```python
from build123d import *

# Parameters (mm, degrees)
BOSS_EXTRUDE1_START = 62.8
SKETCH2_W           = 1.28
SKETCH2_H           = 0.8
BOSS_EXTRUDE1_DEPTH = 6.4
BOSS_EXTRUDE2_START = 65.6
SKETCH3_W           = 1.28
SKETCH3_H           = 6.4
BOSS_EXTRUDE2_DEPTH = 0.8
BOSS_EXTRUDE3_START = 65.2
SKETCH4_W           = 1.8
SKETCH4_H           = 0.9
BOSS_EXTRUDE3_DEPTH = 1.6


with BuildPart() as part:
    # Sketch1 → Revolve1 (revolve)
    with BuildSketch(Plane.XY.offset(66), mode=Mode.PRIVATE) as revolve1_sk:
        Polygon((-58.2, 20.3), (-59.4, 20.3), (-59.4, 18), (-61, 18), (-61, 23.6), (-60.6, 24), (-59.4, 24), (-59.4, 21), (-58.2, 21), align=None)
    revolve(revolve1_sk.sketch.rotate(Axis((-66, 18, 66), (1, 0, 0)), 90), axis=Axis((-66, 18, 66), (1, 0, 0)))


with BuildPart() as body_2:
    # Sketch2 → Boss-Extrude1 (new body)
    with BuildSketch(Plane.XY.offset(BOSS_EXTRUDE1_START)):
        with Locations((-58.74, 18)):
            Rectangle(SKETCH2_W, SKETCH2_H)
    extrude(amount=BOSS_EXTRUDE1_DEPTH)


with BuildPart() as part_1:
    add(part.part)

    # Combine1: cut body 2
    add(body_2.part, mode=Mode.SUBTRACT)


with BuildPart() as body_2_2:
    # Sketch3 → Boss-Extrude2 (new body)
    with BuildSketch(Plane.XY.offset(BOSS_EXTRUDE2_START)):
        with Locations((-58.74, 18)):
            Rectangle(SKETCH3_W, SKETCH3_H)
    extrude(amount=BOSS_EXTRUDE2_DEPTH)


with BuildPart() as part_2:
    add(part_1.part)

    # Combine2: cut body 2 2
    add(body_2_2.part, mode=Mode.SUBTRACT)


with BuildPart() as body_2_3:
    # Sketch4 → Boss-Extrude3 (new body)
    with BuildSketch(Plane.XY.offset(BOSS_EXTRUDE3_START)):
        with Locations((-60.2, 12.35)):
            Rectangle(SKETCH4_W, SKETCH4_H)
    extrude(amount=BOSS_EXTRUDE3_DEPTH)


with BuildPart() as part_3:
    add(part_2.part)

    # Combine3: cut body 2 3
    add(body_2_3.part, mode=Mode.SUBTRACT)


solid = part_3.part
```
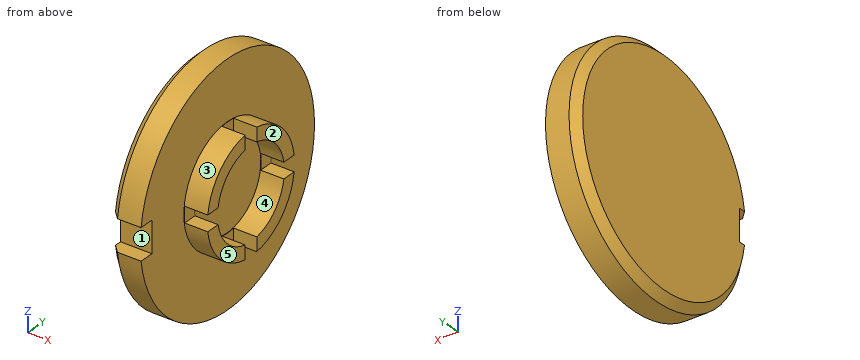
The listing builds one solid part. Answer for the finished solid, in the listing's coordinates (mm). Face numbers are marked on the shaded views. A direction names the side the tool comes from. Give positions to 0.01 mm unless a question says otherwise; leave off trailing zeros. Order: outer loops, then holes, each group sorted by start corner. A loop starts at its lowest first (then second) coordinate and runs counter-clockwise, first axis right, second up. Notation, with made-up numbers: (-29, 2) -> (8, 2) arc R19 ccw to (8, 38) -> close; hole circle Ø3 at (27, 23.5). An arc over 180 degrees is marked (long way). One line per item, written item: value.
1) Find section A-A, the plane x = -58.45. Determine the outline of the cut face in (y, z), plus the area to 3 significant figures.
Reported:
outline: (15.03, 65.6) arc R3 ccw to (17.6, 63.03) -> (17.6, 63.74) arc R2.3 cw to (15.74, 65.6) -> close; (15.03, 66.4) -> (15.74, 66.4) arc R2.3 cw to (17.6, 68.26) -> (17.6, 68.97) arc R3 ccw to start; (18.4, 63.03) arc R3 ccw to (20.97, 65.6) -> (20.26, 65.6) arc R2.3 cw to (18.4, 63.74) -> close; (18.4, 68.26) arc R2.3 cw to (20.26, 66.4) -> (20.97, 66.4) arc R3 ccw to (18.4, 68.97) -> close
area: 9.41 mm^2
2) Flat-ended cylindrical pins translate along their axes: P1, Ø1.5, axis at x = -60, z = 64, coming from the -Y side; P2, Ø1.4, axis at y = 17.5, z = 65.5, coming from the +X side; P3, Ø5, axis at y = 17.5, z = 64.5, coming from the +X side; P4, Ø0.5, axis at x = -60, z = 65.5, coming from the -Y side. Find the tip coordinate at first contact, or state that the pin passes through.
Reported:
P1: stops at y = 12.13
P2: stops at x = -59.4
P3: stops at x = -58.2
P4: stops at y = 12.8
3) Find section D-D, the plane x = -59.9. Determine the outline of the cut face in (y, z).
Reported:
outline: (12.05, 65.2) arc R6 ccw (long way) to (12.05, 66.8) -> (12.8, 66.8) -> (12.8, 65.2) -> close
4) A tool of negligible diameter and unlimited length cuts with its end or side. For the marked faces 4 and 5, from which of +Z, -Z, +X, -X, +Y, -Y can it reach the whole face along a straight path? Write none if from no direction.
Reported:
face 4: +X
face 5: +Z, -Z, +X, +Y, -Y
5) Find the intervals of material crossed by line 1 (X direction, y = 15.5, z = 63.75); line 2 (Y direction, x = -58.6, z = 67.75); line 3 (Y direction, x = -60.8, z = 68), in increasing order.
Reported:
line 1: x = -61 to -59.4
line 2: y = 15.56 to 16.51, 19.49 to 20.44
line 3: y = 12.56 to 23.44
6) Determine the mould class of the marked faces 1, 2 and 3 for opening direction Z: pulls with the +Z half, pulls with the -Z half, needs draft (parallel to the pull), parting line crosses it, or undercut.
Reported:
face 1: undercut
face 2: needs draft
face 3: parting line crosses it
